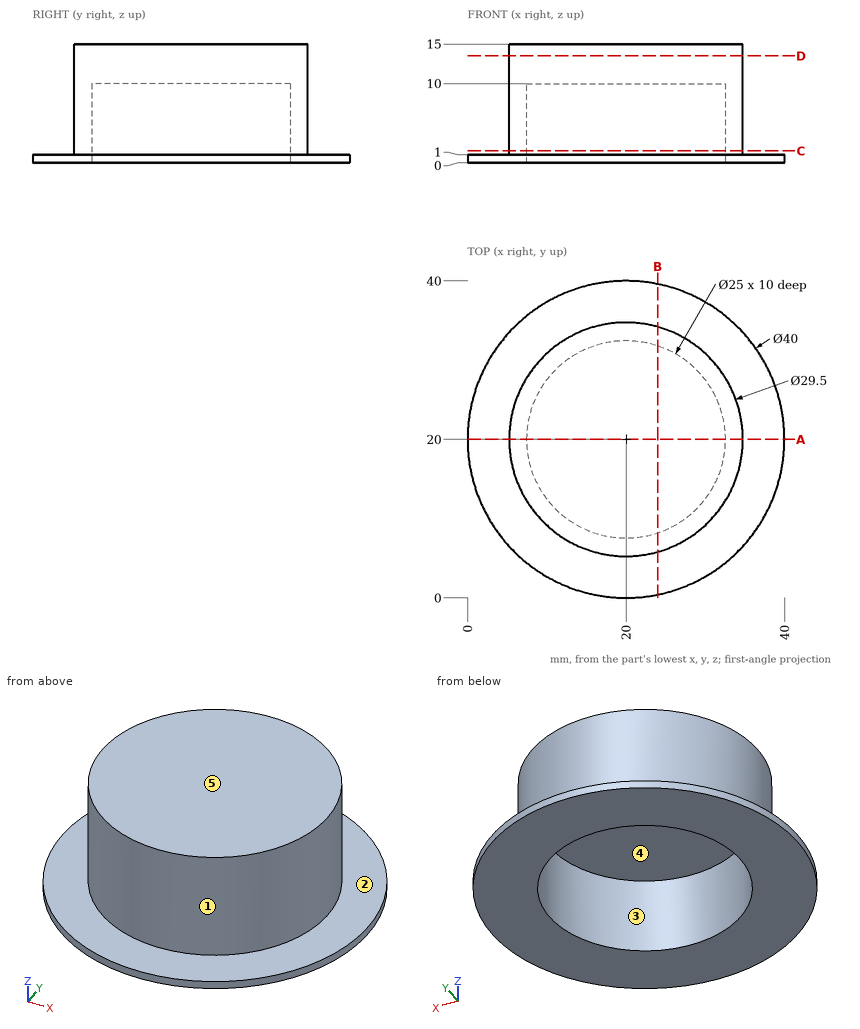
Job drawing, mm, ordinate dimensions from the low corner. One solid piece. A direction names the side the tool comes from. Coordinates: 2 decimals unless noted, no trailing zeros. Write each loop counter-clockwise with the first axis right and the second up, starting at its lowest first coordinate (ties: lowest second). Pieces come first, ordered by that corner, then holes. Notation, with made-up numbers: (36, 52.5) -> (47, 52.5) arc R14 ccw to (47, 76.5) -> close; hole circle Ø8 at (-1, 4.25). An arc over 180 degrees is marked (long way). Use CSV: the item, a comma, the result in double quotes. Start each with the question number.
Item 1: Wall check: probe 1 along Y at (x, z) = (20, 7.25); probe 2 along Y at (x, z) = (10.5, 8.75); probe 3 along Z at (x, y) = (18.5, 28). Give the ranges that are in metal, low to high.
Item 2: Drop flat-ended pins along their axis: P1, Ø1, axis at y = 7, z = 4, coming from the -X side; P2, Ø2, axis at x = 22.5, z = 10.5, coming from the +Y side; P3, Ø8, axis at x = 19.5, z = 9.5, coming from the -Y side. Give the stop position or say it passes through.
Item 3: Band-saw the part on D-D, the plane z = 13.5. Write the cut outline in (x, y), plus the area to 3 significant figures.
Item 4: Tool access for the marked faces 4 and 5: list every direction of +Z, -Z, +X, -X, +Y, -Y with a clear straight run to the whole face (end or side of a thin tool).
Item 5: Band-saw the part on B-B, the plane x = 24. Write the cut outline in (y, z), plus the area to 3 significant figures.
Item 6: Band-saw the part on C-C, the plane z = 1.5. Write the cut outline in (x, y), plus the area to 3 significant figures.
Item 7: Two-plate mould, pull along X, no slides. Class the marked faces 1, 2 and 3: +X half, -X half, draft (parallel to the pull), parting line (faces both ways), or undercut.
Item 8: Band-saw the part on A-A, the plane y = 20. Write the cut outline in (x, z), plus the area to 3 significant figures.
Response values:
1,probe 1,"y = 5.25 to 7.5, 32.5 to 34.75"
1,probe 2,"y = 8.72 to 11.88, 28.12 to 31.28"
1,probe 3,"z = 10 to 15"
2,P1,"stops at x = 12.17"
2,P2,"stops at y = 34.67"
2,P3,"stops at y = 5.25"
3,outline,"circle Ø29.5 at (20, 20)"
3,area,"683 mm2"
4,face 4,"-Z"
4,face 5,"+Z, +X, -X, +Y, -Y"
5,outline,"(0.4, 0) -> (8.16, 0) -> (8.16, 10) -> (31.84, 10) -> (31.84, 0) -> (39.6, 0) -> (39.6, 1) -> (34.2, 1) -> (34.2, 15) -> (5.8, 15) -> (5.8, 1) -> (0.4, 1) -> close"
5,area,"200 mm2"
6,outline,"circle Ø29.5 at (20, 20); hole circle Ø25 at (20, 20)"
6,area,"193 mm2"
7,face 1,"parting line"
7,face 2,"draft"
7,face 3,"undercut"
8,outline,"(0, 0) -> (7.5, 0) -> (7.5, 10) -> (32.5, 10) -> (32.5, 0) -> (40, 0) -> (40, 1) -> (34.75, 1) -> (34.75, 15) -> (5.25, 15) -> (5.25, 1) -> (0, 1) -> close"
8,area,"203 mm2"
